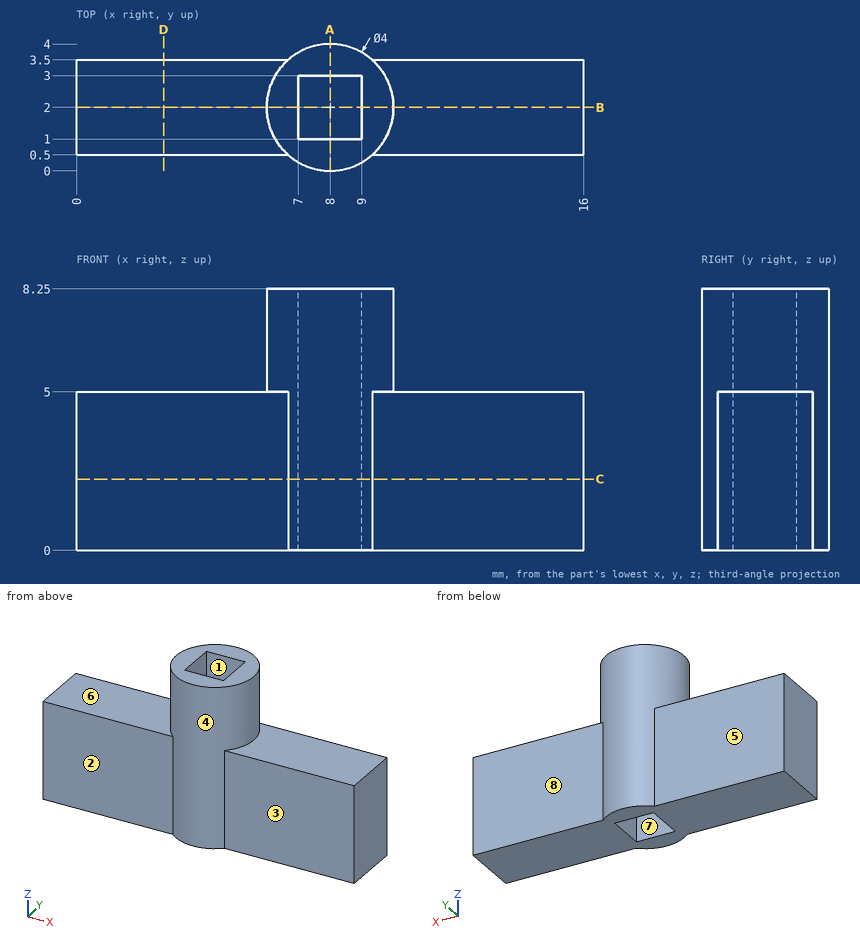
Print and shaded views of the part. All mm, measured from the part's lowest x, y and z. A direction names the side the tool comes from. Give positions to 0.01 mm unless a question says otherwise; leave off trailing zeros. Loops run counter-clockwise (first coordinate to the right, second up) from the corner with the lowest first, then second, coordinate; pieces in that order, holes last.
1) Saw through at A-A (x = 8). Write the cut outline in (y, z), plus the area to 3 significant figures.
2) Pull direction Y, two halves, no side cores. Call the marked faces 6, 7 and 8: +Y half, -Y half, draft (parallel to the pull), parting line (faces both ways), or undercut.
3) Saw through at D-D (x = 2.75). Write the cut outline in (y, z).
4) Tool access for the marked faces 1, 2, 3, 4 and 5: list every direction of +Z, -Z, +X, -X, +Y, -Y with a clear straight run to the whole face (end or side of a thin tool).
5) Wall check: line 1 (X direction, y = 2.6, z = 3.5); line 2 (X direction, y = 2.1, z = 5.25); line 3 (Z direction, x = 11.25, y = 1.1). Give the ranges that are in metal, low to high.
6) Saw through at B-B (y = 2). Write the cut outline in (x, z), plus the area to 3 significant figures.
7) Flat gauge pins, fed straight in: pin 1 Ø4 at (x, z) = (2, 2.5) entering from -Y; pin 2 Ø4 at (x, z) = (10.5, 4.5) entering from +Y; pin 3 Ø2.5 at (x, z) = (3.5, 3.5) entering from +Y. Where does each tip first touch, or does it go through?
8) Saw through at C-C (z = 2.25). Write the cut outline in (x, y), plus the area to 3 significant figures.
Answer block:
1. outline: (0, 0) - (1, 0) - (1, 8.25) - (0, 8.25) - close; (3, 0) - (4, 0) - (4, 8.25) - (3, 8.25) - close
1. area: 16.5 mm2
2. face 6: draft
2. face 7: undercut
2. face 8: +Y half
3. outline: (0.5, 0) - (3.5, 0) - (3.5, 5) - (0.5, 5) - close
4. face 1: +Z, -Z
4. face 2: +Z, -Z, -X, -Y
4. face 3: +Z, -Z, +X, -Y
4. face 4: +Z
4. face 5: +Z, -Z, -X, +Y
5. line 1: x = 0 to 7, 9 to 16
5. line 2: x = 6 to 7, 9 to 10
5. line 3: z = 0 to 5
6. outline: (0, 0) - (7, 0) - (7, 8.25) - (6, 8.25) - (6, 5) - (0, 5) - close; (9, 0) - (16, 0) - (16, 5) - (10, 5) - (10, 8.25) - (9, 8.25) - close
6. area: 76.5 mm2
7. pin 1: stops at y = 0.5
7. pin 2: stops at y = 3.94
7. pin 3: stops at y = 3.5
8. outline: (0, 0.5) - (6.68, 0.5) arc R2 ccw to (9.32, 0.5) - (16, 0.5) - (16, 3.5) - (9.32, 3.5) arc R2 ccw to (6.68, 3.5) - (0, 3.5) - close; hole (7, 1) - (9, 1) - (9, 3) - (7, 3) - close
8. area: 45.8 mm2
